For this review, take the finished solid that the model builds, in its own axes (mm). A direction names the side the tool comes from. Round coordinates to 2 decimals unless told otherwise and drop trailing zeros. Order: outer loops, then holes, each group sorted by start corner. A loop starts at its lowest first (then second) coordinate and runs counter-clockwise, first axis right, second up. Notation, with made-up numbers: (82.5, -31) - (104.5, -31) arc R28 cw to (104.5, -8) - close; hole circle Ø10 at (65, -14.75). An arc over 180 degrees is marked (long way). Write each question's results on one line, items separated by ' | '. Start each with the question number.
(1) Take a section at A-A, the plane y = -36. Give the boundary of the cut face in (x, z), plus the area to 3 significant figures.
(2) For faces 1 (the flat face through (82, 0, 12)), 2 (the flat face through (82, -37, -75.281)), list the 3-axis set-ups (+Z, -Z, +X, -X, +Y, -Y) from which the entire face can be reached by the end or side of a thin tool; tool diameter is ignored.
(3) Take a section at B-B, the plane x = 103. Give the boundary of the cut face in (y, z), plus the area to 3 significant figures.
(4) Draft analysis for pull direction Z (two halves, no side actions). For faces 3 (the flat face through (82, -37, 96.719)), 4 (the flat face through (82, -35, -79.281)), 5 (the flat face through (82, -35, 100.719)), state which applies: pulls with the +Z half, pulls with the -Z half, needs draft (parallel to the pull), parting line crosses it, or undercut.
(5) Insertion check: pin 1 Ø1.5 at (x, z) = (54, -15.5) entering from -Y. The pin has a flat end and moves straight along its axis. Give the tip position at first contact, or say it passes through.
(6) Take a section at C-C, the plane z = 30.5. Give the boundary of the cut face in (x, y), plus the area to 3 significant figures.
(7) For L1, parallel to Z at x = 28, y = -35; L2, parallel to X at y = -40.5, z = 70; L3, parallel to Y at x = 108, z = -60, list the stretches that pass through material, from the lowest coordinate up. Write a range as from..to.
```python
from build123d import *

# Parameters (mm, degrees)
F0_W     = 130
F0_H     = 180
F1_DEPTH = 70
F2_W     = 122
F2_H     = 172
F3_DEPTH = 66
F4_R     = 3


with BuildPart() as f1:
    # F0 (on Front) → F1 (new body)
    with BuildSketch(Plane.XZ):
        with Locations((83.118406, 10.718986)):
            Rectangle(F0_W, F0_H)
    extrude(amount=F1_DEPTH)

    # F2 (on face) → F3 (cut)
    with BuildSketch(Plane.XZ.offset(70)):
        with Locations((83.118406, 10.718986)):
            Rectangle(F2_W, F2_H)
    extrude(amount=-F3_DEPTH, mode=Mode.SUBTRACT)

    # F4
    f4_edges = [f1.edges().sort_by_distance(p)[0] for p in [
        (18.118406, -35, 100.718986),
        (148.118406, -35, 100.718986),
        (18.118406, -35, -79.281014),
        (148.118406, -35, -79.281014),
    ]]
    fillet(f4_edges, radius=F4_R)


solid = f1.part
```
Results below:
1) outline: (18.12, -76.28) arc R3 ccw to (21.12, -79.28) - (145.12, -79.28) arc R3 ccw to (148.12, -76.28) - (148.12, 97.72) arc R3 ccw to (145.12, 100.72) - (21.12, 100.72) arc R3 ccw to (18.12, 97.72) - close; hole (22.12, -75.28) - (144.12, -75.28) - (144.12, 96.72) - (22.12, 96.72) - close | area: 2,410 mm^2
2) face 1: +Z, -Z, +X, -X, +Y | face 2: -Y
3) outline: (-70, -79.28) - (0, -79.28) - (0, 100.72) - (-70, 100.72) - (-70, 96.72) - (-4, 96.72) - (-4, -75.28) - (-70, -75.28) - close | area: 1,250 mm^2
4) face 3: undercut | face 4: pulls with the -Z half | face 5: pulls with the +Z half
5) pin 1: stops at y = -4
6) outline: (18.12, -70) - (22.12, -70) - (22.12, -4) - (144.12, -4) - (144.12, -70) - (148.12, -70) - (148.12, 0) - (18.12, 0) - close | area: 1,050 mm^2
7) L1: z = -79.28..-75.28, 96.72..100.72 | L2: x = 18.12..22.12, 144.12..148.12 | L3: y = -4..0
